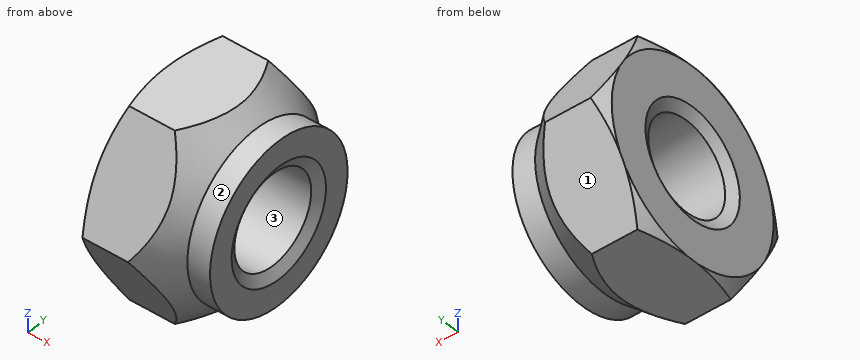
Autodesk Inventor part; units mm, degrees
ref_plane "Work Plane1" through (9.8107, 0, 0) normal (0, 0, 1) x (-1, 0, 0)
ref_plane "YZ Plane" through (0, 0, 0) normal (1, 0, 0) x (0, 1, 0)
ref_plane "XZ Plane" through (0, 0, 0) normal (0, 1, 0) x (-1, 0, 0)
sketch "Esquisse1" plane through (0, 0, 0) normal (1, 0, 0) x (0, 1, 0)
  line L0 (-3.4641, 0) -> (-1.7321, 3)
  line L1 (-1.7321, 3) -> (1.7321, 3)
  line L2 (1.7321, 3) -> (3.4641, 0)
  line L3 (3.4641, 0) -> (1.7321, -3)
  line L4 (1.7321, -3) -> (-1.7321, -3)
  line L5 (-1.7321, -3) -> (-3.4641, 0)
  point P0 (0, 0)
  point P1 (0, 0)
  dimension "d0" = 6.9282
extrude "Corps" add sketch "Esquisse1" along normal blind 3.5
sketch "Esquisse2" plane through (0, 0, 0) normal (-1, 0, 0) x (0, 0, 1)
  line L0 (0, -4.8497) -> (0, 4.8497)
  line L1 (-4.2, 0) -> (4.2, 0)
  point P0 (0, 0)
hole "Filetage" at (0, 0, 0) direction (1, 0, 0) diameter 2.85 end through all
chamfer "Chanfrein1" distance 0.3248 angle 30 1 edges at (0, 0, -1.425) measured on face at (0, -2.123, -1.2698)
chamfer "Chanfrein2" distance 0.3248 angle 30 1 edges at (3.5, 0, -1.425) measured on face at (3.5, -2.123, -1.2698)
sketch "Esquisse3" plane through (0, 0, 0) normal (0, 0, 1) x (1, 0, 0)
  line L0 (0, 1.7321) -> (0, 3.4641)
  line L1 (0, 3.4641) -> (3.5, 3.4641)
  line L2 (3.5, 1.7321) -> (3.5, 3.4641)
  line L3 (-0.7, 0) -> (4.2, 0)
  line L4 (0.2679, 3.4641) -> (0, 3)
  line L5 (3.5, 2.55) -> (2.7894, 2.55)
  line L6 (2.7894, 2.55) -> (1.7, 3.4641)
  dimension "d3" = 30
  dimension "d5" = 6
  dimension "d6" = 5.1
  dimension "d8" = 50
  dimension "d9" = 1.7
revolve "Chanfrein3" cut sketch "Esquisse3" angle 360 about axis through (-10, 0, 0) along (1, 0, 0)
ref_plane "Work Plane1" through (9.8107, 0, 0) normal (0, 0, 1) x (-1, 0, 0)
equation "\"d0\" = 1.1547 * SW"
equation "\"d1\" = KOH"
equation "\"d3\" = ANG1"
equation "\"d5\" = SW0"
equation "\"d6\" = SW1"
equation "\"d8\" = ANG2"
equation "\"d9\" = KOH1"
equation "\"d10\" = -0.5 * GD1 + 0.5 * NND"
equation "\"d39\" = -0.5 * GD1 + 0.5 * NND"
equation "\"d12\" = -0.5 * GD1 + 0.5 * NND"
equation "\"d40\" = -0.5 * GD1 + 0.5 * NND"
equation "\"ANG1\" = 30deg"
equation "\"ANG2\" = 50deg"
equation "\"NND\" = 3.5"
equation "\"KOH\" = 3.5"
equation "\"SW\" = 6"
equation "\"SW0\" = SW"
equation "\"SW1\" = 0.85 * SW"
equation "\"KOH1\" = 1.7"
equation "\"GUL\" = 0.541266 * PTC"
equation "\"THREADDIA\" = 3.5"
equation "\"TOA\" = 30deg"
equation "\"PTC\" = 0.6"
equation "\"E0\" = 1.155 * SW"
equation "\"GAL\" = 0.541266 * PTC"
properties part number "ANSI B18.16.3M - Property Class 5 and 10 - Metric M3.5 x 0.6 Type de métal" material "Acier, doux"
Verification items for the finished model (mm, model axes). Face numbers are marked on the shaded views. Give positions to 0.01 mm unless a question says otherwise; leave off trailing zeros. Loops run counter-clockwise (first coordinate to the right, second up) from the corner with the lowest first, then second, coordinate; pieces in that order, holes last.
1. Section check A-A, the plane x = 3.2. Enter the section's corners in (y, z) (3 decimals), then the cut area to 3 significant figures.
2. Go/stop test with a flat-tipped pin: pin 1 Ø1.5 at (x, z) = (2, -1) entering from +Y. Record where the tip stops, or that it passes through.
3. Thickness scan on line 1 (Z direction, x = 0.4, y = 0) (3 decimals); line 2 (Z direction, x = 2.7, y = 0) (3 decimals); line 3 (Y direction, x = 1.7, z = -0.2). Record the ranges inside material, lowest first.
4. Section check C-C, the plane x = 2.5. Enter the section's corners in (y, z) (3 decimals), then the cut area to 3 significant figures.
5. Mould release check, pull along Y, two halves, no side actions. Record for the marked faces 1, 2 and 3: released by +Y, released by -Y, zero draft, split by the parting line, or undercut.
Geometry says:
1. outline: circle Ø5.1 at (0, 0); hole circle Ø2.85 at (0, 0)
1. area: 14.0 mm2
2. pin 1: stops at y = 3.31
3. line 1: z = -3 to -1.425, 1.425 to 3
3. line 2: z = -2.625 to -1.425, 1.425 to 2.625
3. line 3: y = -3.35 to -1.41, 1.41 to 3.35
4. outline: circle Ø5.586 at (0, 0); hole circle Ø2.85 at (0, 0)
4. area: 18.1 mm2
5. face 1: released by +Y
5. face 2: split by the parting line
5. face 3: undercut
